Verification items for the finished model (mm, model axes). A direction names the side the tool comes from. Round coordinates to 2 decimals unless told otherwise and drop trailing zeros. Write each loop counter-clockwise with the first axis right and the second up, starting at its lowest first coordinate (ties: lowest second). Pieces come first, ordered by that corner, then holes. Notation, with made-up numbers: M 24.25,47.25 L 38.25,47.25 A19 ccw 38.25,79.25 Z; hole C -13.75,83.5 d8. An arc over 180 degrees is marked long. Use a Markdown table: item, result. Add a question column.
from build123d import *

# Parameters (mm, degrees)
BOSS_EXTRUDE1_DEPTH = 70
SKETCH2_R           = 2.2
CUT_EXTRUDE1_DEPTH  = 5.3
FILLET1_R           = 1
SKETCH4_R           = 1.7
CUT_EXTRUDE3_DEPTH  = 10
SKETCH5_R           = 1.75
BOSS_EXTRUDE2_DEPTH = 3
CHAMFER1_SIZE       = 1


with BuildPart() as part:
    # Sketch1 → Boss-Extrude1 (new body)
    with BuildSketch(Plane.XY):
        with BuildLine():
            Line((49, 24), (49, 18.5))
            ThreePointArc((49, 18.5), (49.878679656, 16.378679656), (52, 15.5))
            Line((52, 15.5), (53, 15.5))
            ThreePointArc((53, 15.5), (55.121320344, 14.621320344), (56, 12.5))
            Line((56, 12.5), (56, -12.5))
            ThreePointArc((56, -12.5), (55.121320344, -14.621320344), (53, -15.5))
            Line((53, -15.5), (52, -15.5))
            ThreePointArc((52, -15.5), (49.878679656, -16.378679656), (49, -18.5))
            Line((49, -18.5), (49, -24))
            Line((49, -24), (56, -24))
            ThreePointArc((56, -24), (58.121320344, -23.121320344), (59, -21))
            Line((59, -21), (59, 21))
            ThreePointArc((59, 21), (58.121320344, 23.121320344), (56, 24))
            Line((56, 24), (49, 24))
        make_face()
    extrude(amount=BOSS_EXTRUDE1_DEPTH)

    # Sketch2 → Cut-Extrude1 (cut)
    with BuildSketch(Plane(origin=(0, 0, 0), x_dir=(-1, 0, 0), z_dir=(0, 0, -1))):
        with Locations((-54, -19)):
            Circle(SKETCH2_R)
        with Locations((-54, 19)):
            Circle(SKETCH2_R)
    cut_extrude1 = extrude(amount=-CUT_EXTRUDE1_DEPTH, mode=Mode.SUBTRACT)

    # Mirror1: Cut-Extrude1 across plane
    add(cut_extrude1.mirror(Plane(origin=(0, 0, 35), x_dir=(1, 0, 0), z_dir=(0, 0, -1))), mode=Mode.SUBTRACT)

    # Fillet1
    fillet1_edges = [part.edges().sort_by_distance(p)[0] for p in [
        (49, 24, 35),
    ]]
    fillet(fillet1_edges, radius=FILLET1_R)

    # Sketch4 → Cut-Extrude3 (cut)
    with BuildSketch(Plane(origin=(59, 0, 0), x_dir=(0, 0, -1), z_dir=(1, 0, 0))):
        with Locations(Location((-42, 0, 0), (0, 0, 90))):
            Circle(SKETCH4_R)
        with Locations(Location((-31.5, 6.062177826, 0), (0, 0, 90))):
            Circle(SKETCH4_R)
        with Locations(Location((-31.5, -6.062177826, 0), (0, 0, 90))):
            Circle(SKETCH4_R)
        with BuildLine():
            Line((-64, -5), (-64, 5))
            ThreePointArc((-64, 5), (-60, 9), (-56, 5))
            Line((-56, 5), (-56, -5))
            ThreePointArc((-56, -5), (-60, -9), (-64, -5))
        make_face()
    extrude(amount=-CUT_EXTRUDE3_DEPTH, mode=Mode.SUBTRACT)

    # Sketch5 → Boss-Extrude2 (add)
    with BuildSketch(Plane.XZ.offset(24)):
        with BuildLine():
            Line((49, 2.5), (42, 2.5))
            ThreePointArc((42, 2.5), (39.878679656, 3.378679656), (39, 5.5))
            Line((39, 5.5), (39, 64.5))
            ThreePointArc((39, 64.5), (39.878679656, 66.621320344), (42, 67.5))
            Line((42, 67.5), (49, 67.5))
            Line((49, 67.5), (49, 2.5))
        make_face()
        with Locations((44, 62.5)):
            Circle(SKETCH5_R, mode=Mode.SUBTRACT)
        with Locations(Location((44, 7.5, 0), (0, 0, 180))):
            Circle(SKETCH5_R, mode=Mode.SUBTRACT)
    extrude(amount=-BOSS_EXTRUDE2_DEPTH)

    # Chamfer1
    chamfer1_edges = [part.edges().sort_by_distance(p)[0] for p in [
        (49, -21, 35),
        (49, -22.5, 67.5),
        (49, -22.5, 2.5),
    ]]
    chamfer(chamfer1_edges, length=CHAMFER1_SIZE)


solid = part.part
1. Cross-section at A-A on z = 31.5. Enter the section's corners in (x, y), plus the area to 3 significant figures.
2. Cross-section at C-C on z = 60. Enter the section's corners in (x, y).
3. Scan lines: line 1 along Z through (x, y) = (44, -21.55); line 2 along Y through (x, z) = (54, 2.7); line 3 along Y through (x, z) = (51.75, 53). Record each from-to range of solid material in increasing order. Write a range as from..to.
4. Cross-section at D-D on y = 0. Enter the section's corners in (x, z), plus the area to 3 significant figures.
5. Access from +Z, -Z, +X, -X, +Y, -Y to the whole of each face (thin tool, end or side, straight path). Record for faces 4 (the flat face through (49, 21, 35)), 5 (the cylindrical face through (56.198, -18.903, 2.613)), 6 (the cylindrical face through (55.14, -14.6, 34.51)), 7 (the cylindrical face through (56.198, -18.903, 67.387)), 8 (the flat face through (58, 0, 64)).
6. Depth check by flat-ended pin: pin 1 Ø4 at (x, z) = (44, 62.5) entering from +Y; pin 2 Ø3.5 at (x, y) = (46, -22.5) entering from +Z; pin 3 Ø2.5 at (x, y) = (44, -22) entering from -Z; pin 4 Ø6 at (x, y) = (51, 3) entering from -Z. Enter the tip coordinate at first touch or a pass-through.
7. Release check for a two-part mould opening along Z. For faces 1 (the flat face through (54, -19, 64.7)), 2 (the cylindrical face through (49.9, -16.36, 34.51)), 3 (the cylindrical face through (42.383, -22.521, 8.17)) record: +Z half, -Z half, draft (parallel to the pull), parting line (faces both ways), or undercut.
8. Cross-section at B-B on x = 44. Enter the section's corners in (y, z).
Answer:
| question | item | result |
|---|---|---|
| 1 | outline | M 39,-24 L 56,-24 A3 ccw 59,-21 L 59,-7.76 L 56,-7.76 L 56,-12.5 A3 cw 53,-15.5 L 52,-15.5 A3 ccw 49,-18.5 L 49,-20 L 48,-21 L 39,-21 Z; M 49,18.5 A3 ccw 52,15.5 L 53,15.5 A3 cw 56,12.5 L 56,7.76 L 59,7.76 L 59,21 A3 ccw 56,24 L 50,24 A1 ccw 49,23 Z; M 56,-4.36 L 59,-4.36 L 59,4.36 L 56,4.36 Z |
| 1 | area | 269 mm^2 |
| 2 | outline | M 39,-24 L 56,-24 A3 ccw 59,-21 L 59,-9 L 56,-9 L 56,-12.5 A3 cw 53,-15.5 L 52,-15.5 A3 ccw 49,-18.5 L 49,-20 L 48,-21 L 39,-21 Z; M 49,18.5 A3 ccw 52,15.5 L 53,15.5 A3 cw 56,12.5 L 56,9 L 59,9 L 59,21 A3 ccw 56,24 L 50,24 A1 ccw 49,23 Z |
| 3 | line 1 | z = 2.5..5.75, 9.25..60.75, 64.25..67.5 |
| 3 | line 2 | y = -24..-21.2, -16.8..-15.33, 15.33..16.8, 21.2..24 |
| 3 | line 3 | y = -24..-15.51, 15.51..24 |
| 4 | outline | M 56,0 L 59,0 L 59,40.3 L 56,40.3 Z; M 56,43.7 L 59,43.7 L 59,56 L 56,56 Z; M 56,64 L 59,64 L 59,70 L 56,70 Z |
| 4 | area | 176 mm^2 |
| 5 | face 4 | +Z, -Z, -X, +Y |
| 5 | face 5 | -Z |
| 5 | face 6 | +Z, -Z, -X |
| 5 | face 7 | +Z |
| 5 | face 8 | +X, -X |
| 6 | pin 1 | stops at y = -21 |
| 6 | pin 2 | stops at z = 67.5 |
| 6 | pin 3 | stops at z = 2.5 |
| 6 | pin 4 | passes through |
| 7 | face 1 | +Z half |
| 7 | face 2 | draft |
| 7 | face 3 | undercut |
| 8 | outline | M -24,2.5 L -21,2.5 L -21,5.75 L -24,5.75 Z; M -24,9.25 L -21,9.25 L -21,60.75 L -24,60.75 Z; M -24,64.25 L -21,64.25 L -21,67.5 L -24,67.5 Z |
